Check sheet for the modelled part. Datum: model origin and axes. Units: mm. Give positions to 0.01 mm unless a question says otherwise; leave off trailing zeros. Order: outer loops, then holes, each group sorted by start corner. A loop starts at its lowest first (then second) coordinate and runs counter-clockwise, first axis right, second up. Notation, with made-up numbers: (74.25, 32) - (107.25, 32) arc R23 ccw to (107.25, 53) - close; hole circle Ø6 at (11, 44.5). An arc over 180 degrees is marked (long way). Answer in a Markdown table with one row per item.
Autodesk Inventor part; units mm, degrees
ref_plane "YZ Plane" through (0, 0, 0) normal (1, 0, 0) x (0, 1, 0)
ref_plane "XZ Plane" through (0, 0, 0) normal (0, 1, 0) x (-1, 0, 0)
ref_plane "XY Plane" through (0, 0, 0) normal (0, 0, 1) x (1, 0, 0)
sketch "Sketch1" plane through (0, 0, 0) normal (0, 0, 1) x (1, 0, 0)
  line L0 (0, 0) -> (0, 127)
  line L1 (0, 127) -> (152.4, 127)
  line L2 (152.4, 127) -> (152.4, 0)
  line L3 (152.4, 0) -> (0, 0)
  circle A0 centre (25.4, 120.65) radius 1.905
  line L4 (0, 120.65) -> (152.4, 120.65) construction
  circle A1 centre (141.2875, 117.475) radius 1.5875
  circle A2 centre (141.2875, 9.525) radius 1.5875
  dimension "d0" = 127
  dimension "d1" = 152.4
  dimension "d4" = 3.81
  dimension "d5" = 6.35
  dimension "d6" = 25.4
extrude "Extrusion1" add sketch "Sketch1" along normal blind 3.175
properties part number "Wheel Shield 2" material "Polycarbonate, Clear"
(1) Thickness scan on L1, parallel to Y at x = 25.4, z = 1.3 (3 decimals); L2, parallel to X at y = 120.65, z = 1.5 (3 decimals); L3, parallel to Y at x = 24, z = 0.7. Record the ranges inside material, lowest first.
Geometry says:
| item | result |
|---|---|
| L1 | 0 to 118.745, 122.555 to 127 |
| L2 | 0 to 23.495, 27.305 to 152.4 |
| L3 | 0 to 119.36, 121.94 to 127 |
(2) Mould release check, pull along Y, two halves, no side actions. Record for faces 1 (the flat face through (75, 127, 2)), 2 (the flat face through (0, 63, 2)), 3 (the cylindrical face through (142.802, 116.998, 1.565)): pulls with the +Y half, pulls with the -Y half, needs draft (parallel to the pull), parting line crosses it, or undercut.
Geometry says:
| item | result |
|---|---|
| face 1 | pulls with the +Y half |
| face 2 | needs draft |
| face 3 | undercut |
(3) Cross-section at B-B, the plane y = 120.65. Record the cut outline in (x, z) (3 decimals), then the cut area to 3 significant figures.
Geometry says:
| item | result |
|---|---|
| outline | (0, 0) - (23.495, 0) - (23.495, 3.175) - (0, 3.175) - close; (27.305, 0) - (152.4, 0) - (152.4, 3.175) - (27.305, 3.175) - close |
| area | 472 mm² |
(4) Gauge pin test, flat end, axial feed: P1, Ø6, axis at x = 25.4, y = 120.65, coming from the +Z side (3 decimals). Record the tip position at first contact, or that the pin passes through.
Geometry says:
| item | result |
|---|---|
| P1 | z = 3.175 |
(5) Cross-section at A-A, the plane x = 25.4. Record the cut outline in (y, z) (3 decimals), then the cut area to 3 significant figures.
Geometry says:
| item | result |
|---|---|
| outline | (0, 0) - (118.745, 0) - (118.745, 3.175) - (0, 3.175) - close; (122.555, 0) - (127, 0) - (127, 3.175) - (122.555, 3.175) - close |
| area | 391 mm² |
